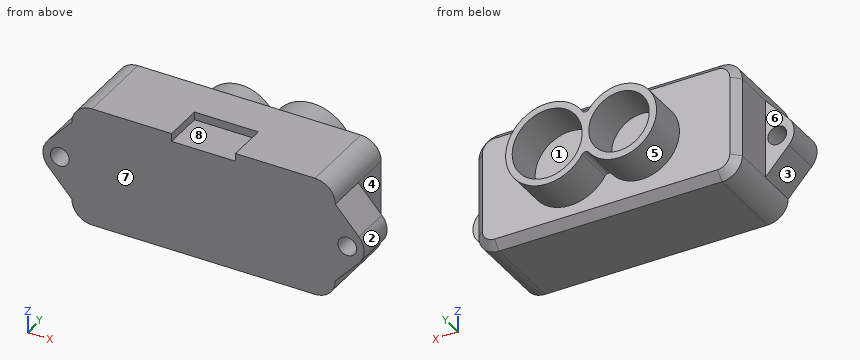
from build123d import *

# Parameters (mm, degrees)
BOSS_EXTRUDE1_DEPTH = 5.5
SKETCH2_R           = 1.175
BOSS_EXTRUDE2_DEPTH = 5
CHAMFER1_SIZE       = 1
SKETCH3_R           = 3.793643162
SKETCH3_R_2         = 4.381481481
BOSS_EXTRUDE3_DEPTH = 5
SKETCH4_W           = 8
SKETCH4_H           = 5
CUT_EXTRUDE1_DEPTH  = 1


with BuildPart() as part:
    # Sketch1 → Boss-Extrude1 (new body, symmetric)
    with BuildSketch(Plane(origin=(0, 0, 0), x_dir=(1, 0, 0), z_dir=(0, 1, 0))):
        with BuildLine():
            Line((-13.96, 7.5), (13.96, 7.5))
            ThreePointArc((13.96, 7.5), (15.756051224, 6.756051224), (16.5, 4.96))
            Line((16.5, 4.96), (16.5, -4.96))
            ThreePointArc((16.5, -4.96), (15.756051224, -6.756051224), (13.96, -7.5))
            Line((13.96, -7.5), (-13.96, -7.5))
            ThreePointArc((-13.96, -7.5), (-15.756051224, -6.756051224), (-16.5, -4.96))
            Line((-16.5, -4.96), (-16.5, 4.96))
            ThreePointArc((-16.5, 4.96), (-15.756051224, 6.756051224), (-13.96, 7.5))
        make_face()
    extrude(amount=BOSS_EXTRUDE1_DEPTH, both=True)

    # Sketch2 → Boss-Extrude2 (add)
    with BuildSketch(Plane.XZ.offset(5.5)):
        with BuildLine():
            Line((-16.5, 4.96), (-19.451582405, 1.706700282))
            ThreePointArc((-19.451582405, 1.706700282), (-20.110419428, 0), (-19.451582405, -1.706700282))
            Line((-19.451582405, -1.706700282), (-16.5, -4.96))
            Line((-16.5, -4.96), (16.5, -4.96))
            Line((16.5, -4.96), (19.451582406, -1.706700282))
            ThreePointArc((19.451582406, -1.706700282), (20.110419428, 0), (19.451582405, 1.706700282))
            Line((19.451582405, 1.706700282), (16.5, 4.96))
            Line((16.5, 4.96), (-15.93880857, 4.96))
            Line((-15.93880857, 4.96), (-16.5, 4.96))
        make_face()
        with Locations((-18, 0)):
            Circle(SKETCH2_R, mode=Mode.SUBTRACT)
        with Locations((18, 0)):
            Circle(SKETCH2_R, mode=Mode.SUBTRACT)
    extrude(amount=-BOSS_EXTRUDE2_DEPTH)

    # Chamfer1
    chamfer1_edges = [part.edges().sort_by_distance(p)[0] for p in [
        (-15.756051224, 5.5, -6.756051224),
        (-16.5, 5.5, 0),
        (-15.756051224, 5.5, 6.756051224),
        (0, 5.5, 7.5),
        (15.756051224, 5.5, 6.756051224),
        (16.5, 5.5, 0),
        (15.756051224, 5.5, -6.756051224),
        (0, 5.5, -7.5),
    ]]
    chamfer(chamfer1_edges, length=CHAMFER1_SIZE)

    # Sketch3 → Boss-Extrude3 (add)
    with BuildSketch(Plane(origin=(0, 5.5, 0), x_dir=(1, 0, 0), z_dir=(0, 1, 0))):
        with BuildLine():
            ThreePointArc((-0.706356838, 2.774575924), (-9.2, 0), (-0.706356838, -2.774575924))
            ThreePointArc((-0.706356838, -2.774575924), (-0.287091072, -2.569989708), (0.118518519, -2.800467823))
            ThreePointArc((0.118518519, -2.800467823), (9.7, 0), (0.118518519, 2.800467823))
            ThreePointArc((0.118518519, 2.800467823), (-0.287091072, 2.569989708), (-0.706356838, 2.774575924))
        make_face()
        with Locations((-4.5, 0)):
            Circle(SKETCH3_R, mode=Mode.SUBTRACT)
        with Locations((4.5, 0)):
            Circle(SKETCH3_R_2, mode=Mode.SUBTRACT)
    extrude(amount=BOSS_EXTRUDE3_DEPTH)

    # Sketch4 → Cut-Extrude1 (cut)
    with BuildSketch(Plane.XY.offset(7.5)):
        with Locations((0, -3)):
            Rectangle(SKETCH4_W, SKETCH4_H)
    extrude(amount=-CUT_EXTRUDE1_DEPTH, mode=Mode.SUBTRACT)


solid = part.part
Design review of the part built by this model. Coordinates are the model's own, in mm. Face numbers are marked on the shaded views. A direction names the side the tool comes from. Round coordinates to 2 decimals unless told otherwise and drop trailing zeros. Write each loop counter-clockwise with the first axis right and the second up, starting at its lowest first coordinate (ties: lowest second). Pieces come first, ordered by that corner, then holes. Notation, with made-up numbers: (57, 50) -> (103, 50) arc R15 cw to (103, 70) -> close; hole circle Ø8 at (83.25, 5). An arc over 180 degrees is marked (long way). One line per question, with ' | ' between items.
(1) Wall thickness on line 1 (X direction, y = 9.35, z = 0); line 2 (Z direction, x = 4.5, y = 6.55); line 3 (X direction, y = 8.5, z = -3.25): over which ranges is each line inside the solid? List them lowest first. Write a range as [from, to].
Result sheet:
line 1: [-9.2, -8.29], [-0.71, 0.12], [8.88, 9.7] | line 2: [-5.2, -4.38], [4.38, 5.2] | line 3: [-7.9, -6.46], [-2.54, -1.1], [0.44, 1.56], [7.44, 8.56]
(2) Take a section at C-C, the plane y = 0.75. State the section outline as (x, z) points.
Result sheet:
outline: (-16.5, -4.96) arc R2.54 ccw to (-13.96, -7.5) -> (13.96, -7.5) arc R2.54 ccw to (16.5, -4.96) -> (16.5, 4.96) arc R2.54 ccw to (13.96, 7.5) -> (-13.96, 7.5) arc R2.54 ccw to (-16.5, 4.96) -> close
(3) Machinability: for the marked faces 4, 5, 6, 7 and 8, which of the approach directions +Z, -Z, +X, -X, +Y, -Y give a long, thin tool a straight path to every point of the face, cutting with its end or side? Answer none if there is none.
Result sheet:
face 4: +Z, -Z, +X, +Y | face 5: +Y | face 6: +Z, -Z, -X, +Y | face 7: +Z, -Z, +X, -X, -Y | face 8: +Z, -Y
(4) Take a section at A-A, the plane x = 4.5. State the section outline as (y, z) points.
Result sheet:
outline: (-5.5, -7.5) -> (4.5, -7.5) -> (5.5, -6.5) -> (5.5, -5.2) -> (10.5, -5.2) -> (10.5, -4.38) -> (5.5, -4.38) -> (5.5, 4.38) -> (10.5, 4.38) -> (10.5, 5.2) -> (5.5, 5.2) -> (5.5, 6.5) -> (4.5, 7.5) -> (-5.5, 7.5) -> close
(5) Take a section at D-D, the plane x = -18. State the section outline as (y, z) points (3 decimals), and give its area (3 significant figures).
Result sheet:
outline: (-5.5, -3.307) -> (-0.5, -3.307) -> (-0.5, -1.175) -> (-5.5, -1.175) -> close; (-5.5, 1.175) -> (-0.5, 1.175) -> (-0.5, 3.307) -> (-5.5, 3.307) -> close | area: 21.3 mm2
(6) Draft analysis for pull direction X (two halves, no side actions). For the marked faces 1, 2 and 3, state which applies: released by +X, released by -X, zero draft, split by the parting line, or undercut.
Result sheet:
face 1: undercut | face 2: released by +X | face 3: released by -X
(7) Take a section at B-B, the plane z = 0. State how many separate pieces and enclosed holes the cut face has, and give its area (3 significant figures).
Result sheet:
separate pieces: 3 | enclosed holes: 0 | area: 387 mm2
(8) Insertion check: P1, Ø2, axis at x = 18, z = 0, coming from the +Y side; P2, Ø2, axis at y = -2.5, z = 4.5, coming from the +X side; P3, Ø1, axis at y = 4.5, z = -6, coming from the -X side; P4, Ø1.5, axis at y = 8.5, z = -4.5, coming from the +X side. Each pin has a flat end and moves straight along its axis. Give the tip position at first contact, or say it passes through.
Result sheet:
P1: through | P2: x = 17.82 | P3: x = -16.44 | P4: x = 8.1
